from build123d import *

# Parameters (mm, degrees)
SKETCH1_W             = 76
SKETCH1_H             = 62
BOSS_EXTRUDE1_DEPTH   = 2
SKETCH2_W             = 82
SKETCH2_H             = 68
BOSS_EXTRUDE2_DEPTH   = 8
SKETCH3_W             = 45
SKETCH3_H             = 12.8
CUT_EXTRUDE1_DEPTH    = 11
SKETCH4_R             = 1.6
CUT_EXTRUDE2_DEPTH    = 11
SKETCH5_R             = 3.1
CUT_EXTRUDE3_DEPTH    = 3
SKETCH9_OUTSIDE_W     = 105.4
SKETCH9_OUTSIDE_H     = 91.4
SKETCH9_OUTSIDE_W_2   = 75.6
SKETCH9_OUTSIDE_H_2   = 61.6
CUT_EXTRUDE5_DEPTH    = 3
CUT_EXTRUDE6_DEPTH    = 3
SKETCH11_W            = 66
SKETCH11_H            = 54
CUT_EXTRUDE7_DEPTH    = 7
CHAMFER2_SIZE         = 2
CHAMFER2_SIZE2        = 0.352653961
CHAMFER2_PART_2_SIZE  = 2
CHAMFER2_PART_2_SIZE2 = 0.352653961
CHAMFER3_SIZE         = 1
CHAMFER3_SIZE2        = 1.732050808


with BuildPart() as part:
    # Sketch1 → Boss-Extrude1 (new body)
    with BuildSketch(Plane(origin=(0, 0, 0), x_dir=(1, 0, 0), z_dir=(0, 1, 0))):
        Rectangle(SKETCH1_W, SKETCH1_H)
    extrude(amount=BOSS_EXTRUDE1_DEPTH)

    # Sketch2 → Boss-Extrude2 (add)
    with BuildSketch(Plane(origin=(0, 2, 0), x_dir=(1, 0, 0), z_dir=(0, 1, 0))):
        Rectangle(SKETCH2_W, SKETCH2_H)
    extrude(amount=BOSS_EXTRUDE2_DEPTH)

    # Sketch3 → Cut-Extrude1 (cut, through all)
    with BuildSketch(Plane.XZ):
        Rectangle(SKETCH3_W, SKETCH3_H)
    extrude(amount=-CUT_EXTRUDE1_DEPTH, mode=Mode.SUBTRACT)

    # Sketch4 → Cut-Extrude2 (cut, through all)
    with BuildSketch(Plane(origin=(0, 10, 0), x_dir=(1, 0, 0), z_dir=(0, 1, 0))):
        with Locations(Location((-35.408866178, 29.363450001, 0), (0, 0, 270))):  # turned: the seam where the file's is
            Circle(SKETCH4_R)
        with Locations(Location((35.408866178, 29.363450001, 0), (0, 0, 270))):  # turned: the seam where the file's is
            Circle(SKETCH4_R)
        with Locations(Location((35.408866178, -29.363450001, 0), (0, 0, 270))):  # turned: the seam where the file's is
            Circle(SKETCH4_R)
        with Locations(Location((-35.408866178, -29.363450001, 0), (0, 0, 270))):  # turned: the seam where the file's is
            Circle(SKETCH4_R)
    extrude(amount=-CUT_EXTRUDE2_DEPTH, mode=Mode.SUBTRACT)

    # Sketch5 → Cut-Extrude3 (cut)
    with BuildSketch(Plane(origin=(0, 10, 0), x_dir=(1, 0, 0), z_dir=(0, 1, 0))):
        with Locations(Location((-35.408866178, 29.363450001, 0), (0, 0, 270))):  # turned: the seam where the file's is
            Circle(SKETCH5_R)
        with Locations(Location((35.408866178, 29.363450001, 0), (0, 0, 270))):  # turned: the seam where the file's is
            Circle(SKETCH5_R)
        with Locations(Location((35.408866178, -29.363450001, 0), (0, 0, 270))):  # turned: the seam where the file's is
            Circle(SKETCH5_R)
        with Locations(Location((-35.408866178, -29.363450001, 0), (0, 0, 270))):  # turned: the seam where the file's is
            Circle(SKETCH5_R)
    extrude(amount=-CUT_EXTRUDE3_DEPTH, mode=Mode.SUBTRACT)

    # Sketch9 outside → Cut-Extrude5 (cut)
    with BuildSketch(Plane.XZ):
        Rectangle(SKETCH9_OUTSIDE_W, SKETCH9_OUTSIDE_H)
        Rectangle(SKETCH9_OUTSIDE_W_2, SKETCH9_OUTSIDE_H_2, mode=Mode.SUBTRACT)
    extrude(amount=-CUT_EXTRUDE5_DEPTH, mode=Mode.SUBTRACT)

    # Sketch10 → Cut-Extrude6 (cut)
    with BuildSketch(Plane.XZ):
        Polygon((-37.8, -30.8), (-31.8, -30.8), (-37.8, -24.8), align=None)
        Polygon((-37.8, 24.8), (-37.8, 30.8), (-31.8, 30.8), align=None)
        Polygon((37.8, 30.8), (37.8, 24.8), (31.8, 30.8), align=None)
        Polygon((37.8, -30.8), (31.8, -30.8), (37.8, -24.8), align=None)
    extrude(amount=-CUT_EXTRUDE6_DEPTH, mode=Mode.SUBTRACT)

    # Sketch11 → Cut-Extrude7 (cut)
    with BuildSketch(Plane.XZ):
        Rectangle(SKETCH11_W, SKETCH11_H)
    extrude(amount=-CUT_EXTRUDE7_DEPTH, mode=Mode.SUBTRACT)

    # Chamfer2
    chamfer2_edges = [part.edges().sort_by_distance(p)[0] for p in [
        (37.8, 0, 0),
    ]]
    chamfer2_side = [part.faces().sort_by_distance(p)[0] for p in [
        (37.8, 1.5, 0),
    ]]
    chamfer(chamfer2_edges, length=CHAMFER2_SIZE, length2=CHAMFER2_SIZE2, reference=chamfer2_side[0])

    # Chamfer2 part 2
    chamfer2_part_2_edges = [part.edges().sort_by_distance(p)[0] for p in [
        (-37.8, 0, 0),
    ]]
    chamfer2_part_2_side = [part.faces().sort_by_distance(p)[0] for p in [
        (-37.8, 1.5, 0),
    ]]
    chamfer(chamfer2_part_2_edges, length=CHAMFER2_PART_2_SIZE, length2=CHAMFER2_PART_2_SIZE2, reference=chamfer2_part_2_side[0])

    # Chamfer3
    chamfer3_edges = [part.edges().sort_by_distance(p)[0] for p in [
        (0, 0, -30.8),
        (0, 0, 30.8),
    ]]
    chamfer3_side = [part.faces().sort_by_distance(p)[0] for p in [
        (-35.357643735, 0, 25.870950059),
    ]]
    chamfer(chamfer3_edges, length=CHAMFER3_SIZE, length2=CHAMFER3_SIZE2, reference=chamfer3_side[0])


solid = part.part
Build history of the part. All positions in model axes, mm. A direction names the side the tool comes from. Give positions to 0.01 mm unless a question says otherwise; leave off trailing zeros. Order: outer loops, then holes, each group sorted by start corner. A loop starts at its lowest first (then second) coordinate and runs counter-clockwise, first axis right, second up. Notation, with made-up numbers: M -5.5,-12 L 48.5,-12 A25 ccw 48.5,3 Z; hole C 14.5,-35 d5. An arc over 180 degrees is marked long. Use one line per item in the form item = value.
1) Two-plate mould, pull along X, no slides. Class faces 1 (the face through (34, 7, 31)), 2 (the face through (0, 0, 29)), 3 (the face through (-36.2, 1.5, 26.4)), 4 (the face through (0, 8, -6.4)): released by +X, released by -X, zero draft, split by the parting line, or undercut.
Calculated:
face_1 = undercut
face_2 = zero draft
face_3 = released by -X
face_4 = undercut
2) Saw through at D-D (x = -28). Give the cut face in (y, z), plus the area to 3 significant figures.
Calculated:
outline = M 0,-29.8 L 1.73,-30.8 L 3,-30.8 L 3,-34 L 10,-34 L 10,34 L 3,34 L 3,30.8 L 1.73,30.8 L 0,29.8 L 0,27 L 7,27 L 7,-27 L 0,-27 Z
area = 281 mm2
3) Saw through at C-C (y = 8.5). Give the cut face in (x, z).
Calculated:
outline = M -41,-34 L 41,-34 L 41,34 L -41,34 Z; hole C -35.41,-29.36 d6.2; hole C -35.41,29.36 d6.2; hole M -22.5,-6.4 L 22.5,-6.4 L 22.5,6.4 L -22.5,6.4 Z; hole C 35.41,-29.36 d6.2; hole C 35.41,29.36 d6.2
4) Saw through at B-B (z = -19.5). Give the cut face in (x, y), plus the area to 3 significant figures.
Calculated:
outline = M -41,3 L -37.8,3 L -37.8,2 L -37.45,0 L -33,0 L -33,7 L 33,7 L 33,0 L 37.45,0 L 37.8,2 L 37.8,3 L 41,3 L 41,10 L -41,10 Z
area = 338 mm2
5) Saw through at A-A (x = 0). Give the cut face in (y, z), plus the area to 3 significant figures.
Calculated:
outline = M 0,-29.8 L 1.73,-30.8 L 3,-30.8 L 3,-34 L 10,-34 L 10,-6.4 L 7,-6.4 L 7,-27 L 0,-27 Z; M 0,27 L 7,27 L 7,6.4 L 10,6.4 L 10,34 L 3,34 L 3,30.8 L 1.73,30.8 L 0,29.8 Z
area = 243 mm2
6) Probe probe 1 along Z at (x, y) = (-15.5, 1.75); probe 2 along X at (y, z) = (5, 9.5); probe 3 along Z at (x, y) = (14, 3.5). List the from-to ranges inside material, lowest first.
Calculated:
probe_1 = -30.8 to -27, 27 to 30.8
probe_2 = -41 to -33, 33 to 41
probe_3 = -34 to -27, 27 to 34
7) Tool access for faces 5 (the face through (-38.159, 8.521, -27.933)), 6 (the face through (36.2, 1.5, 26.4)), 7 (the face through (0, 3, -27)): list every direction of +Z, -Z, +X, -X, +Y, -Y with a clear straight run to the whole face (end or side of a thin tool).
Calculated:
face_5 = +Y
face_6 = +Z, +X, -Y
face_7 = -Y
8) Drop flat-ended pins along their axis: pin 1 (2 mm diameter, centred on x = -2, z = -23.5, fed in from -Y); pin 2 (3 mm diameter, centred on x = 35.5, z = 28.5, fed in from +Y); pin 3 (2 mm diameter, centred on y = 1.5, z = 17, fed in from +X). Give the stop position or say it passes through.
Calculated:
pin_1 = 7
pin_2 = 7
pin_3 = 37.8
